For this review, take the finished solid that the model builds, in its own axes (mm). A direction names the side the tool comes from. Coordinates: 2 decimals unless noted, no trailing zeros. Loops run counter-clockwise (first coordinate to the right, second up) from the corner with the lowest first, then second, coordinate; pieces in that order, holes last. Notation, with made-up numbers: (-17, -25) - (0, -25) arc R22 cw to (0, -7) - close; hole circle Ø10 at (8.25, 37). An arc over 180 degrees is marked (long way). One line per item, written item: value. Start each with the question number.
1. The part is to be moulded in two halves that separate along X. For faces 1 (the face through (84, 1, 46)), 2 (the face through (75, -11.5, 46)), 3 (the face through (89, -2, 48)), say which applies: released by +X, released by -X, zero draft, split by the parting line, or undercut.
2. Take a section at D-D, the plane y = -5.5. State the section outline as (x, z) points.
3. Take a section at A-A, the plane y = 0. State the section outline as (x, z) points, and give its area (3 significant figures).
4. To check wall thickness, follow line 1 (X direction, y = 1.25, z = 53.5); line 2 (Y direction, x = 70, z = 50); line 3 (Y direction, x = 68, z = 52.25). State the ranges of each line that lie inside material, in increasing order. Write a range as from..to.
5. Take a section at C-C, the plane x = 75. State the section outline as (y, z) points, and give its area (3 significant figures).
6. Take a section at B-B, the plane z = 46. State the section outline as (x, y) points.
7. Insertion check: pin 1 (1 mm diameter, centred on x = 80.5, y = -6.5, fed in from -Z); pin 2 (2 mm diameter, centred on y = -1.5, z = 54, fed in from -X); pin 3 (2.5 mm diameter, centred on y = 0, z = 44, fed in from -X). Each pin has a flat end and moves straight along its axis. Give the tip position at first contact, or say it passes through.
8. For faces 4 (the face through (79, 9, 46)), 5 (the face through (86.535, 4.957, 45.349)), 6 (the face through (79, -10, 46)), list the 3-axis set-ups (+Z, -Z, +X, -X, +Y, -Y) from which the entire face can be reached by the end or side of a thin tool; tool diameter is ignored.
```python
from build123d import *

# Parameters (mm, degrees)
CYLINDER203_R             = 5
CYLINDER203_DEPTH         = 5
CYLINDER204_R             = 2.5
CYLINDER204_DEPTH         = 20
CYLINDER001_R             = 11.5
CYLINDER001_DEPTH         = 4.5
CYLINDER002_R             = 4
CYLINDER002_DEPTH         = 23
CYLINDER_R                = 8.5
CYLINDER_DEPTH            = 15
FUSION_PLACEMENT_ANGLE    = 90
FUSION041_PLACEMENT_ANGLE = 180


with BuildPart() as cylinder203:
    # Cylinder203 → Cylinder203 (new body)
    with BuildSketch(Plane(origin=(15, 0, 0), x_dir=(0, 0, -1), z_dir=(1, 0, 0))):
        Circle(CYLINDER203_R)
    extrude(amount=CYLINDER203_DEPTH)


with BuildPart() as pinion:
    # Cylinder204 → Cylinder204 (new body)
    with BuildSketch(Plane(origin=(0, 0, 0), x_dir=(0, 0, -1), z_dir=(1, 0, 0))):
        Circle(CYLINDER204_R)
    extrude(amount=CYLINDER204_DEPTH)

    # Fusion040: union Cylinder203
    add(cylinder203.part)


with BuildPart() as pinion_1:
    # Fusion040 placement: moved
    add(pinion.part.moved(Location((-21.5, 54.5, 7.5))))


with BuildPart() as cylinder001:
    # Cylinder001 → Cylinder001 (new body)
    with BuildSketch(Plane.XY.offset(-1)):
        Circle(CYLINDER001_R)
    extrude(amount=CYLINDER001_DEPTH)


with BuildPart() as cylinder002:
    # Cylinder002 → Cylinder002 (new body)
    with BuildSketch(Plane.XY.offset(-5)):
        Circle(CYLINDER002_R)
    extrude(amount=CYLINDER002_DEPTH)


with BuildPart() as differential_pinion:
    # Cylinder → Cylinder (new body)
    with BuildSketch(Plane.XY.offset(-1)):
        Circle(CYLINDER_R)
    extrude(amount=CYLINDER_DEPTH)

    # Fusion: union Cylinder001, Cylinder002
    add(cylinder001.part)
    add(cylinder002.part)


with BuildPart() as differential_pinion_1:
    # Fusion placement: moved
    add(differential_pinion.part.moved(Location((7.5, 48, 7.5))).rotate(Axis((7.5, 48, 7.5), (-1, 0, 0)), FUSION_PLACEMENT_ANGLE))

    # Fusion041: union pinion
    add(pinion_1.part)


with BuildPart() as differential_pinion_2:
    # Fusion041 placement: moved
    add(differential_pinion_1.part.moved(Location((82.5, -54.5, 53.5))).rotate(Axis((82.5, -54.5, 53.5), (0, 1, 0)), FUSION041_PLACEMENT_ANGLE))


solid = differential_pinion_2.part
```
Solutions:
1. face 1: undercut
1. face 2: zero draft
1. face 3: released by +X
2. outline: circle Ø23 at (75, 46)
3. outline: circle Ø17 at (75, 46); (84, 41) - (89, 41) - (89, 43.5) - (104, 43.5) - (104, 48.5) - (89, 48.5) - (89, 51) - (84, 51) - close
3. area: 352 mm2
4. line 1: 71..79
4. line 2: -7.5..7.5
4. line 3: -7.5..-3
5. outline: (-11.5, 42) - (-7.5, 42) - (-7.5, 34.5) - (-3, 34.5) - (-3, 37.5) - (7.5, 37.5) - (7.5, 42) - (11.5, 42) - (11.5, 50) - (7.5, 50) - (7.5, 54.5) - (-3, 54.5) - (-3, 57.5) - (-7.5, 57.5) - (-7.5, 50) - (-11.5, 50) - close
5. area: 346 mm2
6. outline: (63.5, -7.5) - (71, -7.5) - (71, -11.5) - (79, -11.5) - (79, -7.5) - (86.5, -7.5) - (86.5, -5) - (89, -5) - (89, -2.5) - (104, -2.5) - (104, 2.5) - (89, 2.5) - (89, 5) - (84, 5) - (84, -3) - (83.5, -3) - (83.5, 7.5) - (79, 7.5) - (79, 11.5) - (71, 11.5) - (71, 7.5) - (66.5, 7.5) - (66.5, -3) - (63.5, -3) - close
7. pin 1: z = 35.64
7. pin 2: x = 70.18
7. pin 3: x = 66.53
8. face 4: +Y
8. face 5: +X
8. face 6: -Y
